For this review, use the dimensioned drawing (mm, ordinates from the lowest corner) and the shaded views. Coordinates: 2 decimals unless noted, no trailing zeros. Write each loop counter-clockwise with the first axis right and the second up, starting at its lowest first coordinate (ties: lowest second). Pieces come first, ordered by that corner, then holes.
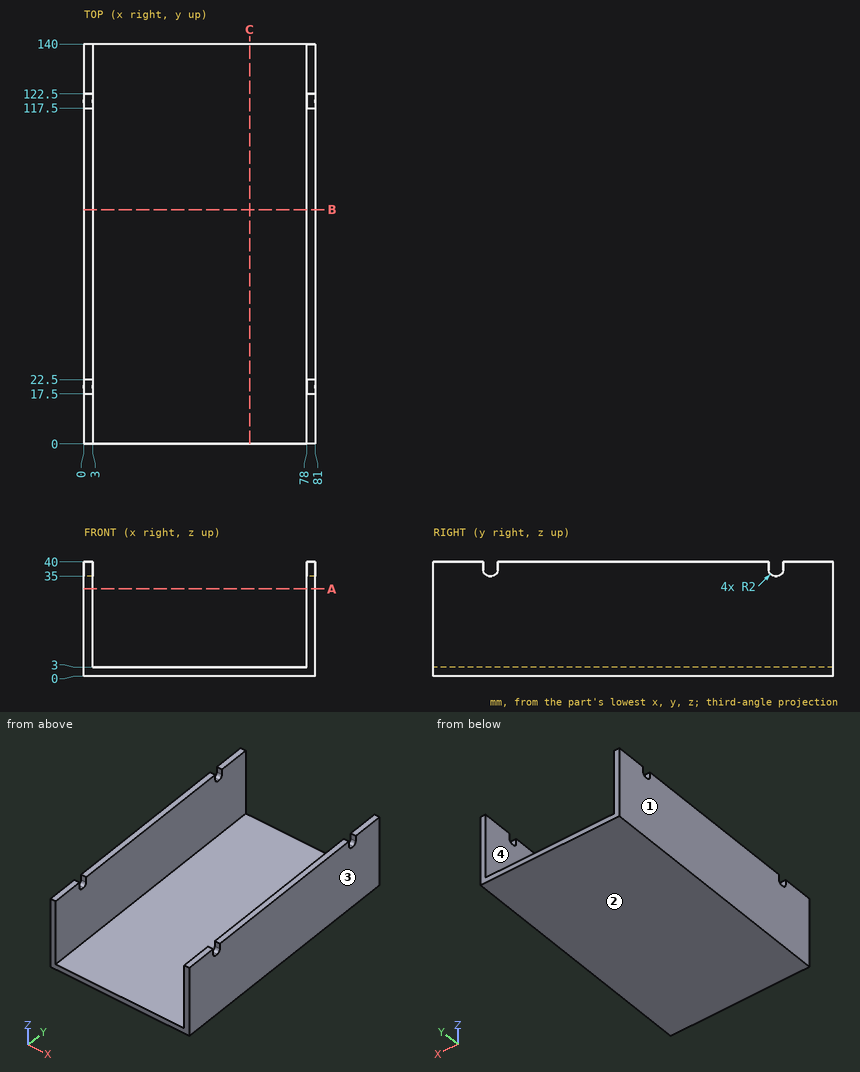
Item 1: Take a section at A-A, the plane z = 30.5. Write out the cut boundary in (x, y).
Solved:
outline: (0, 0) - (3, 0) - (3, 140) - (0, 140) - close; (78, 0) - (81, 0) - (81, 140) - (78, 140) - close
Item 2: To check wall thickness, follow line 1 along X through (y, z) = (46, 16); line 2 along Z through (x, y) = (31, 36). State the ranges of each line that lie inside material, in increasing order.
Solved:
line 1: x = 0 to 3, 78 to 81
line 2: z = 0 to 3
Item 3: For pin 1 (8 mm diameter, centred on x = 49, y = 87, fed in from +Z); pin 2 (5 mm diameter, centred on x = 8.5, z = 7.5, fed in from -Y); pin 3 (0.5 mm diameter, centred on x = 79, y = 120, fed in from +Z), all flat-tipped, find the tip position at first contact; note any pin that passes through.
Solved:
pin 1: stops at z = 3
pin 2: passes through
pin 3: stops at z = 35
Item 4: Take a section at B-B, the plane y = 82. Write out the cut boundary in (x, z), plus the area to 3 significant figures.
Solved:
outline: (0, 0) - (81, 0) - (81, 40) - (78, 40) - (78, 3) - (3, 3) - (3, 40) - (0, 40) - close
area: 465 mm2
Item 5: Mouldability with a two-part tool opening along X and no side actions: class the marked faces 1, 2, 3 and 4 as pulls with the +X half, pulls with the -X half, needs draft (parallel to the pull), parting line crosses it, or undercut.
Solved:
face 1: pulls with the -X half
face 2: needs draft
face 3: pulls with the +X half
face 4: undercut
Item 6: Take a section at C-C, the plane x = 58. Write out the cut boundary in (y, z).
Solved:
outline: (0, 0) - (140, 0) - (140, 3) - (0, 3) - close
